```python
from build123d import *

# Parameters (mm, degrees)
SKETCH_1_W      = 110
SKETCH_1_H      = 110
EXTRUDE_1_DEPTH = 71
SKETCH_2_W      = 110
SKETCH_2_H      = 15
EXTRUDE_3_DEPTH = 10
SKETCH_3_W      = 110
SKETCH_3_H      = 15
EXTRUDE_4_DEPTH = 10


with BuildPart() as part:
    # 草图1 → 凸台-拉伸1 (new body)
    with BuildSketch(Plane(origin=(0, 0, 0), x_dir=(1, 0, 0), z_dir=(0, 1, 0))):
        with Locations((55, 55)):
            Rectangle(SKETCH_1_W, SKETCH_1_H)
    extrude(amount=EXTRUDE_1_DEPTH)

    # 草图2 → 凸台-拉伸3 (add)
    with BuildSketch(Plane.XY):
        with Locations((55, 16.5)):
            Rectangle(SKETCH_2_W, SKETCH_2_H)
    extrude(amount=EXTRUDE_3_DEPTH)

    # 草图3 → 凸台-拉伸4 (add)
    with BuildSketch(Plane(origin=(0, 0, -110), x_dir=(-1, 0, 0), z_dir=(0, 0, -1))):
        with Locations((-55, 16.5)):
            Rectangle(SKETCH_3_W, SKETCH_3_H)
    extrude(amount=EXTRUDE_4_DEPTH)


solid = part.part
```
The listing builds one solid part. Answer for the finished solid, in the listing's coordinates (mm). A direction names the side the tool comes from. Round coordinates to 2 decimals unless told otherwise and drop trailing zeros. Loops run counter-clockwise (first coordinate to the right, second up) from the corner with the lowest first, then second, coordinate; pieces in that order, holes last. Notation, with made-up numbers: (75.25, 21) - (132.25, 21) arc R18 cw to (132.25, 29) - close; hole circle Ø11 at (48, 80). An arc over 180 degrees is marked (long way). Use one line per item in the form item = value. Start each with the question number.
1. Given pin 1 Ø10 at (x, y) = (63.5, 33.5) entering from -Z; pin 2 Ø14 at (x, y) = (72, 43.5) entering from +Z; pin 3 Ø8 at (x, z) = (46.5, 5.5) entering from -Y, each flat-ended and moving along its own axis, determine where each tip first touches the part or whether it passes through.
2. A tool of negligible diameter and unlimited length cuts with its end or side. For faces 1 (the face through (54, 24, 5)), 2 (the face through (54, 9, 5)), 3 (the face through (56, 24, -115)), 4 (the face through (56, 9, -115)), from which of +Z, -Z, +X, -X, +Y, -Y can it reach the whole face along a straight path? Write none if from no direction.
3. The part is cut by section A-A on x = 84.5. Determine the outline of the cut face in (y, z).
4. Consider line 1 (Z direction, x = 37.5, y = 49.5); line 2 (Y direction, x = 14.5, z = 1.5). Determine where each line is inside the solid, lowest interval first. Write a range as [from, to].
5. The part is cut by section B-B on y = 33. Determine the outline of the cut face in (x, z).
Geometry check:
q1.pin_1 = -110
q1.pin_2 = 0
q1.pin_3 = 9
q2.face_1 = +Z, +X, -X, +Y
q2.face_2 = +Z, +X, -X, -Y
q2.face_3 = -Z, +X, -X, +Y
q2.face_4 = -Z, +X, -X, -Y
q3.outline = (0, -110) - (9, -110) - (9, -120) - (24, -120) - (24, -110) - (71, -110) - (71, 0) - (24, 0) - (24, 10) - (9, 10) - (9, 0) - (0, 0) - close
q4.line_1 = [-110, 0]
q4.line_2 = [9, 24]
q5.outline = (0, -110) - (110, -110) - (110, 0) - (0, 0) - close
